from build123d import *

# Parameters (mm, degrees)
EXTRUDE_1_DEPTH     = 1
EXTRUDE_START       = 11.5
EXTRUDE_3_DEPTH     = 11.5
EXTRUDE_START_2     = 1
EXTRUDE_4_DEPTH     = 1
FILLET_1_R          = 1
FILLET_2_R          = 1
SKETCH_7_W          = 7.249999999999998
SKETCH_7_H          = 1
CUT_EXTRUDE_1_DEPTH = 1.5
SKETCH1_R           = 0.8
CUT_EXTRUDE1_DEPTH  = 10


with BuildPart() as part:
    # 草图1 → 凸台-拉伸1 (new body)
    with BuildSketch(Plane(origin=(0, 0, 0), x_dir=(1, 0, 0), z_dir=(0, 1, 0))):
        with BuildLine():
            Line((11.995707880639234, -1.030263157894738), (9.275971038533973, -8.032758066524272))
            Line((9.275971038533973, -8.032758066524272), (6.200000000000001, -10.73871500692704))
            ThreePointArc((6.200000000000001, -10.73871500692704), (-11.456106203139957, 4.7452745613271095), (11.977480245984443, 3.2093561592712687))
            Line((11.977480245984443, 3.2093561592712687), (11.995707880639234, -1.030263157894738))
        make_face()
        with BuildLine():
            Line((9.5, 0), (6.733552631578949, -6.701437827642379))
            ThreePointArc((6.733552631578949, -6.701437827642379), (-8.78119439484174, 3.625), (9.5, 0))
        make_face(mode=Mode.SUBTRACT)
    extrude(amount=EXTRUDE_1_DEPTH)

    # 草图2 → 凸台-拉伸3 (add)
    with BuildSketch(Plane(origin=(0, 0, 0), x_dir=(-1, 0, 0), z_dir=(0, -1, 0)).offset(EXTRUDE_START)):
        with BuildLine():
            Line((-11.995707880639236, -1.0302631578947385), (-11.97748024598447, 3.2093561592711763))
            ThreePointArc((-11.97748024598447, 3.2093561592711763), (11.456106203139939, 4.745274561327148), (-6.2, -10.738715006927038))
            Line((-6.2, -10.738715006927038), (-9.275971038533974, -8.032758066524272))
            Line((-9.275971038533974, -8.032758066524272), (-11.995707880639236, -1.0302631578947385))
        make_face()
        with BuildLine():
            Line((-8.045661066301793, -7.353729530394456), (-10.889013517064273, -0.4892694811569148))
            ThreePointArc((-10.889013517064273, -0.4892694811569148), (10.070286904373022, 4.171249412779482), (-8.045661066301793, -7.353729530394456))
        make_face(mode=Mode.SUBTRACT)
    extrude(amount=-EXTRUDE_3_DEPTH)

    # 草图5 → 凸台-拉伸4 (add)
    with BuildSketch(Plane(origin=(0, -11.5, 0), x_dir=(-1, 0, 0), z_dir=(0, -1, 0)).offset(EXTRUDE_START_2)):
        with BuildLine():
            Line((-11.977480245984468, 3.2093561592711772), (-11.995707880639236, -1.0302631578947385))
            Line((-11.995707880639236, -1.0302631578947385), (-9.275971038533974, -8.032758066524272))
            Line((-9.275971038533974, -8.032758066524272), (-6.200000000000009, -10.738715006927029))
            ThreePointArc((-6.200000000000009, -10.738715006927029), (11.456106203139935, 4.745274561327147), (-11.977480245984468, 3.2093561592711772))
        make_face()
        with BuildLine():
            Line((-9.5, 0), (-6.733552631578949, -6.701437827642379))
            ThreePointArc((-6.733552631578949, -6.701437827642379), (8.78119439484174, 3.624999999999999), (-9.5, 0))
        make_face(mode=Mode.SUBTRACT)
    extrude(amount=-EXTRUDE_4_DEPTH)

    # 圆角1
    # the kernel refuses this fillet: 1 mm, written as the material it takes off along each edge
    with BuildSketch(Plane(origin=(11.1530264468926, -12.5, 6.38149703508447), x_dir=(-0.6605044125759205, 0, -0.75082216334345), z_dir=(-0.75082216334345, 0, 0.6605044125759205))) as fillet_1_piece_1:
        with BuildLine():
            CenterArc((FILLET_1_R, -FILLET_1_R), FILLET_1_R, 90, 90)
            Line((0, -FILLET_1_R), (0, 0))
            Line((0, 0), (FILLET_1_R, 0))
        make_face()
    extrude(amount=9.096803728910329, mode=Mode.SUBTRACT)
    with BuildSketch(Plane(origin=(3.36e-15, -12.5, -3.77e-15), x_dir=(0.663902971885599, 0, 0.7478187239709029), z_dir=(0.7478187239709029, 0, -0.663902971885599))) as fillet_1_piece_2:
        with BuildLine():
            CenterArc((12.399999999999997 - FILLET_1_R, -FILLET_1_R), FILLET_1_R, 0, 90)
            Line((12.399999999999997 - FILLET_1_R, 0), (12.399999999999997, 0))
            Line((12.399999999999997, 0), (12.399999999999999, -FILLET_1_R))
        make_face()
    revolve(axis=Axis((3.36e-15, -12.5, -3.77e-15), (0, -1, 0)), revolution_arc=308.1964386657649, mode=Mode.SUBTRACT)
    with BuildSketch(Plane(origin=(11.966731954198387, -12.5, -5.709333054009145), x_dir=(0, 1, 0), z_dir=(0.0042993167144171895, 0, 0.9999907578951863))) as fillet_1_piece_3:
        with BuildLine():
            CenterArc((FILLET_1_R, FILLET_1_R), FILLET_1_R, 180, 90)
            Line((0, FILLET_1_R), (0, 0))
            Line((0, 0), (FILLET_1_R, 0))
        make_face()
    extrude(amount=9.239658500534155, mode=Mode.SUBTRACT)
    with BuildSketch(Plane(origin=(12.900824508619046, -12.5, -1.3001367841226104), x_dir=(7e-17, 1, 3e-17), z_dir=(-0.36204665119192375, 0, 0.9321599768069393))) as fillet_1_piece_4:
        with BuildLine():
            CenterArc((FILLET_1_R, FILLET_1_R), FILLET_1_R, 180, 90)
            Line((-8e-17, FILLET_1_R), (0, 0))
            Line((0, 0), (FILLET_1_R, 0))
        make_face()
    extrude(amount=12.512117107426324, mode=Mode.SUBTRACT)

    # 圆角2
    # the kernel refuses this fillet: 1 mm, written as the material it takes off along each edge
    with BuildSketch(Plane(origin=(11.966731954198387, 1, -5.709333054009236), x_dir=(0, -1, 0), z_dir=(0.004299316714422545, 0, 0.9999907578951863))) as fillet_2_piece_1:
        with BuildLine():
            CenterArc((FILLET_2_R, -FILLET_2_R), FILLET_2_R, 90, 90)
            Line((0, -FILLET_2_R), (0, 0))
            Line((0, 0), (FILLET_2_R, 0))
        make_face()
    extrude(amount=9.239658500534247, mode=Mode.SUBTRACT)
    with BuildSketch(Plane(origin=(6e-17, 1, 1.33e-15), x_dir=(0.6639029718855987, 0, 0.7478187239709033), z_dir=(0.7478187239709033, 0, -0.6639029718855987))) as fillet_2_piece_2:
        with BuildLine():
            CenterArc((12.4 - FILLET_2_R, FILLET_2_R), FILLET_2_R, 270, 90)
            Line((12.4 - FILLET_2_R, 0), (12.4, 0))
            Line((12.4, 0), (12.400000000000002, FILLET_2_R))
        make_face()
    revolve(axis=Axis((6e-17, 1, 1.33e-15), (0, -1, 0)), revolution_arc=308.19643866576433, mode=Mode.SUBTRACT)
    with BuildSketch(Plane(origin=(11.153026446892596, 1, 6.381497035084468), x_dir=(-0.6605044125759212, 0, -0.7508221633434493), z_dir=(-0.7508221633434494, 0, 0.6605044125759213))) as fillet_2_piece_3:
        with BuildLine():
            CenterArc((FILLET_2_R, FILLET_2_R), FILLET_2_R, 180, 90)
            Line((0, FILLET_2_R), (0, 0))
            Line((0, 0), (FILLET_2_R, 0))
        make_face()
    extrude(amount=9.096803728910343, mode=Mode.SUBTRACT)
    with BuildSketch(Plane(origin=(12.900824508619046, 1, -1.3001367841226104), x_dir=(-0.9321599768069392, 0, -0.3620466511919237), z_dir=(-0.36204665119192375, 0, 0.9321599768069393))) as fillet_2_piece_4:
        with BuildLine():
            CenterArc((FILLET_2_R, FILLET_2_R), FILLET_2_R, 180, 90)
            Line((8e-17, FILLET_2_R), (0, 0))
            Line((0, 0), (FILLET_2_R, 0))
        make_face()
    extrude(amount=12.512117107426329, mode=Mode.SUBTRACT)

    # 草图7 → 切除-拉伸1 (cut)
    with BuildSketch(Plane(origin=(8.116776315789474, 0, 3.3507189138211895), x_dir=(-0.3815789473684208, 0, 0.9243362520886044), z_dir=(-0.9243362520886044, 0, -0.3815789473684208))):
        with Locations((0, 0.5)):
            Rectangle(SKETCH_7_W, SKETCH_7_H)
    extrude(amount=-CUT_EXTRUDE_1_DEPTH, mode=Mode.SUBTRACT)

    # Sketch1 → Cut-Extrude1 (cut)
    with BuildSketch(Plane(origin=(-10.219164738912983, -5.75, 7.023437337867946), x_dir=(0.5664062369248344, 0, 0.8241261886220147), z_dir=(-0.8241261886220146, 0, 0.5664062369248343))):
        Circle(SKETCH1_R)
    extrude(amount=-CUT_EXTRUDE1_DEPTH, mode=Mode.SUBTRACT)


solid = part.part
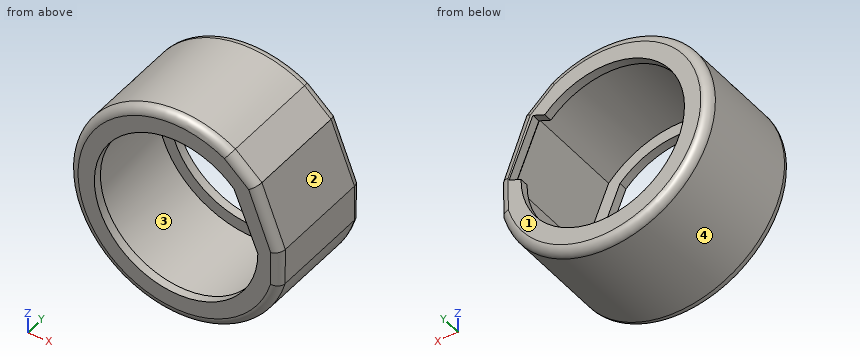
Geometry: final body of the model. Coordinates: model frame, mm. Face numbers are marked on the shaded views. Give positions to 0.01 mm unless a question says otherwise; leave off trailing zeros. Write each loop counter-clockwise with the first axis right and the second up, starting at its lowest first coordinate (ties: lowest second). Pieces come first, ordered by that corner, then holes. Notation, with made-up numbers: M 61.5,46 L 115.5,46 A22 ccw 115.5,76 Z; hole C 45.25,-0.5 d8. An arc over 180 degrees is marked long. Answer in a Markdown table with one row per item. Add a question column.
(1) Ray query, line 1 (X direction, y = -5.5, z = 0); line 2 (Y direction, x = -7.5, z = -6.25); line 3 (Z direction, x = 0, y = -5.5). Return the intervals inside material, ascending.
(2) Section B-B on y = -4. Return loops of the section in (x, z).
(3) First-contact query: pin 1 (4 mm diameter, centred on x = 5, y = -2, fed in from +Z); pin 2 (1.5 mm diameter, centred on y = -4.5, z = 5, fed in from -X). Flat tips, straight axial feed; report the tip coordinate or a pass-through.
(4) Mould query, pull axis Z, two halves, no side actions, for the marked faces 1, 2, 3 and 4. Classes: +Z half, -Z half, draft (parallel to the pull), parting line (faces both ways), or undercut.
(5) Section A-A on x = 0. Return loops of the section in (y, z), and give its area (3 significant figures).
Result set:
| question | item | result |
|---|---|---|
| 1 | line 1 | x = -12.4 to -10.9, 10.9 to 11.99 |
| 1 | line 2 | y = -12.5 to -11.5, 0 to 1 |
| 1 | line 3 | z = -12.4 to -10.9, 10.9 to 12.4 |
| 2 | outline | M 6.2,10.74 A12.4 ccw long 11.98,-3.21 L 12,1.03 L 9.28,8.03 Z; hole M 8.05,7.35 A10.9 ccw long 10.89,0.49 Z |
| 3 | pin 1 | stops at z = 12.03 |
| 3 | pin 2 | stops at x = -11.65 |
| 4 | face 1 | draft |
| 4 | face 2 | +Z half |
| 4 | face 3 | undercut |
| 4 | face 4 | parting line |
| 5 | outline | M -12.5,-11.4 A1 ccw -11.5,-12.4 L 0,-12.4 A1 ccw 1,-11.4 L 1,-9.5 L 0,-9.5 L 0,-10.9 L -11.5,-10.9 L -11.5,-9.5 L -12.5,-9.5 Z; M -12.5,9.5 L -11.5,9.5 L -11.5,10.9 L 0,10.9 L 0,9.5 L 1,9.5 L 1,11.4 A1 ccw 0,12.4 L -11.5,12.4 A1 ccw -12.5,11.4 Z |
| 5 | area | 45.2 mm^2 |
